Input: part model. Units: mm. Frame: model coordinates. Face numbers are marked on the shaded views. A direction names the side the tool comes from. Coordinates: 2 decimals unless noted, no trailing zeros. Write each loop counter-clockwise with the first axis right and the second up, starting at its lowest first coordinate (ties: lowest second). Pieces come first, ordered by that corner, then holes. Notation, with made-up numbers: M 41.5,1 L 87.5,1 A20 cw 87.5,15 Z; hole C -1.75,-36 d8. An arc over 180 degrees is marked long. Use CSV: the item, a comma, the result in double quotes.
```python
from build123d import *

# Parameters (mm, degrees)
F0_W            = 20
F0_H            = 46.5
F1_DEPTH        = 164
F2_W            = 164
F2_H            = 3.1
F3_DEPTH        = 10
F4_W            = 164
F4_H            = 13
F5_DEPTH        = 2
F7_DEPTH        = 46.5
F8_R            = 12.99999
F10_D           = 4
F10_DEPTH       = 20
F10_CSINK_D     = 7.8
F10_CSINK_ANGLE = 90
F10_TIP         = 1.2017212381
F12_DEPTH       = 20
F13_R           = 7.5
F14_DEPTH       = 13
F15_R           = 5.6
F16_DEPTH       = 5
F17_W           = 38
F17_H           = 15.9
F17_H_2         = 11.1
F18_DEPTH       = 12
F20_DEPTH       = 6
F21_W           = 38
F21_H           = 4
F22_DEPTH       = 4
F23_W           = 38
F23_H           = 4
F24_DEPTH       = 4


# Not quite as in the source:
# - a fillet or chamfer is up to 0.001 mm smaller than in the source, because OpenCascade refuses the exact size


with BuildPart() as f1:
    # F0 (on Front) → F1 (new body)
    with BuildSketch(Plane.XZ):
        Rectangle(F0_W, F0_H)
    extrude(amount=F1_DEPTH)

    # F2 (on face) → F3 (cut)
    with BuildSketch(Plane(origin=(-10, 0, 0), x_dir=(0, -1, 0), z_dir=(-1, 0, 0))):
        with Locations((82, 8.7)):
            Rectangle(F2_W, F2_H)
    extrude(amount=-F3_DEPTH, mode=Mode.SUBTRACT)

    # F4 (on face) → F5 (cut)
    with BuildSketch(Plane(origin=(-10, 0, 0), x_dir=(0, -1, 0), z_dir=(-1, 0, 0))):
        with Locations((82, -16.75)):
            Rectangle(F4_W, F4_H)
    extrude(amount=-F5_DEPTH, mode=Mode.SUBTRACT)

    # F6 (on face) → F7 (cut, through all)
    with BuildSketch(Plane.XY.offset(23.25)):
        Polygon((-10, 0), (-10, -20), (10, 0), align=None)
    extrude(amount=-F7_DEPTH, mode=Mode.SUBTRACT)

    # F8 (radius 13 in the source; OpenCascade refuses exactly that, so slightly less here)
    f8_edges = [f1.edges().sort_by_distance(p)[0] for p in [
        (-10, -92, 23.25),
    ]]
    fillet(f8_edges, radius=F8_R)

    # F10
    with Locations(Plane.YZ.offset(10)):
        with Locations((-123, -16.75), (-41, -16.75)):
            CounterSinkHole(F10_D / 2, F10_CSINK_D / 2, depth=F10_DEPTH, counter_sink_angle=F10_CSINK_ANGLE)
            with Locations((0, 0, -(F10_DEPTH + F10_TIP / 2))):  # 118° drill point
                Cone(0, F10_D / 2, F10_TIP, mode=Mode.SUBTRACT)

    # F11 (on face) → F12 (cut, through all)
    with BuildSketch(Plane(origin=(-10, 0, 0), x_dir=(0, -1, 0), z_dir=(-1, 0, 0))):
        with BuildLine():
            Line((63.4057692308, -3.5508088231), (63.4057692308, 0.4508088231))
            ThreePointArc((63.4057692308, 0.4508088231), (59.9090942784, 2.3989538045), (56.5057692308, 0.2919694165))
            Line((56.5057692308, 0.2919694165), (56.5057692308, -3.3919694165))
            ThreePointArc((56.5057692308, -3.3919694165), (59.9090942784, -5.4989538045), (63.4057692308, -3.5508088231))
        make_face()
    extrude(amount=-F12_DEPTH, mode=Mode.SUBTRACT)

    # F13 (on face) → F14 (cut)
    with BuildSketch(Plane(origin=(-10, 0, 0), x_dir=(0, -1, 0), z_dir=(-1, 0, 0))):
        with Locations((60, -1.55)):
            Circle(F13_R)
        with BuildLine():
            Line((63.4057692308, 0.4508088231), (63.4057692308, -3.5508088231))
            ThreePointArc((63.4057692308, -3.5508088231), (59.9090942784, -5.4989538045), (56.5057692308, -3.3919694165))
            Line((56.5057692308, -3.3919694165), (56.5057692308, 0.2919694165))
            ThreePointArc((56.5057692308, 0.2919694165), (59.9090942784, 2.3989538045), (63.4057692308, 0.4508088231))
        make_face(mode=Mode.SUBTRACT)
    extrude(amount=-F14_DEPTH, mode=Mode.SUBTRACT)

    # F15 (on face) → F16 (cut)
    with BuildSketch(Plane.YZ.offset(10)):
        with Locations((-59.9557692308, -1.6294197033)):
            Circle(F15_R)
        with BuildLine():
            ThreePointArc((-56.5057692308, -3.3919694165), (-59.9090942784, -5.4989538045), (-63.4057692308, -3.5508088231))
            Line((-63.4057692308, -3.5508088231), (-63.4057692308, 0.4508088231))
            ThreePointArc((-63.4057692308, 0.4508088231), (-59.9090942784, 2.3989538045), (-56.5057692308, 0.2919694165))
            Line((-56.5057692308, 0.2919694165), (-56.5057692308, -3.3919694165))
        make_face(mode=Mode.SUBTRACT)
    extrude(amount=-F16_DEPTH, mode=Mode.SUBTRACT)

    # F17 (on face) → F18 (cut)
    with BuildSketch(Plane(origin=(-10, 0, 0), x_dir=(0, -1, 0), z_dir=(-1, 0, 0))):
        with Locations((94, -2.3)):
            Rectangle(F17_W, F17_H)
        with Locations((94, -15.8)):
            Rectangle(F17_W, F17_H_2)
    extrude(amount=-F18_DEPTH, mode=Mode.SUBTRACT)

    # F19 (on face) → F20 (cut)
    with BuildSketch(Plane(origin=(-10, 0, 0), x_dir=(0, -1, 0), z_dir=(-1, 0, 0))):
        with BuildLine():
            Line((75, -3.1), (75, 0))
            Line((75, 0), (67.3380855814, 0))
            ThreePointArc((67.3380855814, 0), (67.4594115673, -0.7707830407), (67.5, -1.55))
            ThreePointArc((67.5, -1.55), (67.4594115673, -2.3292169593), (67.3380855814, -3.1))
            Line((67.3380855814, -3.1), (75, -3.1))
        make_face()
    extrude(amount=-F20_DEPTH, mode=Mode.SUBTRACT)

    # F21 (on face) → F22 (cut)
    with BuildSketch(Plane(origin=(2, 0, 0), x_dir=(0, -1, 0), z_dir=(-1, 0, 0))):
        with Locations((94, 3.65)):
            Rectangle(F21_W, F21_H)
    extrude(amount=-F22_DEPTH, mode=Mode.SUBTRACT)

    # F23 (on face) → F24 (cut)
    with BuildSketch(Plane(origin=(2, 0, 0), x_dir=(0, -1, 0), z_dir=(-1, 0, 0))):
        with Locations((94, -19.35)):
            Rectangle(F23_W, F23_H)
    extrude(amount=-F24_DEPTH, mode=Mode.SUBTRACT)


solid = f1.part
```
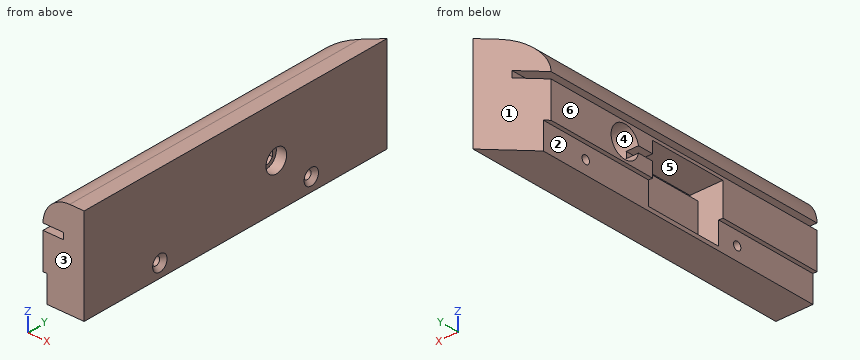
1. Contact query for flat-ended pins moving along their axis: pin 1 Ø3 at (y, z) = (-123, -16.75) entering from -X (3 decimals); pin 2 Ø8 at (x, y) = (-3.5, -33.5) entering from +Z; pin 3 Ø2 at (x, y) = (-9.5, -51.5) entering from -Z; pin 4 Ø6.5 at (x, y) = (-7, -70.5) entering from +Z. Output: stop coordinate, or through.
Resolved:
pin 1,"passes through"
pin 2,"stops at z = 23.01"
pin 3,"stops at z = -10.25"
pin 4,"stops at z = 21.36"
2. Section A-A (x = -1.5). Return loops of the section in (y, z).
Resolved:
outline,"M -164,-23.25 L -11.5,-23.25 L -11.5,7.15 L -164,7.15 Z; M -164,10.25 L -11.5,10.25 L -11.5,22.45 L -164,22.45 Z; hole C -123,-16.75 d4; hole M -113,-21.35 L -75,-21.35 L -75,5.65 L -113,5.65 Z; hole C -60,-1.55 d15; hole C -41,-16.75 d4"
3. Material intervals for line 1 (Y direction, x = -0.25, z = -16.75); line 2 (Z direction, x = 5.5, y = -76); line 3 (Z direction, x = 4.5, y = -123), sorted ascending. Write a range as [from, to].
Resolved:
line 1,"y = [-164, -125], [-121, -113], [-75, -43], [-39, -10.25]"
line 2,"z = [-23.25, -21.35], [-17.35, 1.65], [5.65, 23.25]"
line 3,"z = [-23.25, -18.75], [-14.75, 23.25]"
4. Access query for the marked faces 5 and 6. Directions: +Z, -Z, +X, -X, +Y, -Y. A direction counts if a zero-diameter tool reaches every point of the face in a straight line with its end or side. Return the directions, or none.
Resolved:
face 5,"-X"
face 6,"+Z, -Z, -X, +Y, -Y"
5. Mould query, pull axis Y, two halves, no side actions, for the marked faces 1, 2, 3 and 4. Classes: pulls with the +Y half, pulls with the -Y half, needs draft (parallel to the pull), parting line crosses it, or undercut.
Resolved:
face 1,"pulls with the +Y half"
face 2,"needs draft"
face 3,"pulls with the -Y half"
face 4,"undercut"
